Can you work these out from the model? Positions are in its coordinate system, mm. Face numbers are marked on the shaded views. Give positions to 0.01 mm unless a question says otherwise; leave off trailing zeros. Write each loop counter-clockwise with the first axis right and the second up, starting at its lowest first coordinate (ties: lowest second). Pieces come first, ordered by that corner, then holes. Notation, with made-up numbers: (66, -3) -> (112, -3) arc R11 ccw to (112, 3) -> close; hole circle Ø5 at (36, -19). An arc over 180 degrees is marked (long way). One line per item, written item: value.
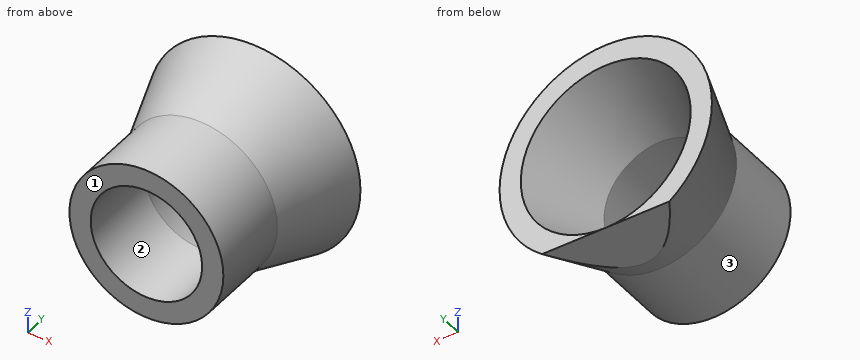
from build123d import *

# Parameters (mm, degrees)
CROQUIS2_R              = 7.25
CROQUIS2_R_2            = 5.25
SALIENTE_EXTRUIR1_DEPTH = 7.5
CORTAR_EXTRUIR1_DEPTH   = 7.5


with BuildPart() as part:
    # Croquis1 → Revolución1 (revolve)
    with BuildSketch(Plane.XY):
        Polygon((-5.25, 0), (-8, 7.5), (-10, 7.5), (-7.25, 0), align=None)
    revolve(axis=Axis((0, 7.5, 0), (0, -1, 0)))

    # Croquis2 → Saliente-Extruir1 (add)
    with BuildSketch(Plane.XZ):
        Circle(CROQUIS2_R)
        Circle(CROQUIS2_R_2, mode=Mode.SUBTRACT)
    extrude(amount=SALIENTE_EXTRUIR1_DEPTH)

    # Croquis4 → Cortar-Extruir1 (cut)
    with BuildSketch(Plane(origin=(0, 7.5, 0), x_dir=(1, 0, 0), z_dir=(0, 1, 0))):
        Polygon((-8.604100246, 8), (8.604100246, 8), (0, 12.592023512), align=None)
    extrude(amount=-CORTAR_EXTRUIR1_DEPTH, mode=Mode.SUBTRACT)


solid = part.part
1) If we section it at A-A (z = 0): Write out the boundary of the cut face in (x, y).
Answer list:
outline: (-10, 7.5) -> (-7.25, 0) -> (-7.25, -7.5) -> (-5.25, -7.5) -> (-5.25, 0) -> (-8, 7.5) -> close; (5.25, -7.5) -> (7.25, -7.5) -> (7.25, 0) -> (10, 7.5) -> (8, 7.5) -> (5.25, 0) -> close
2) Will these pins go through, and if not, where does the flat tip stop? pin 1 (8 mm diameter, centred on y = 2.5, z = 3.5, fed in from -X); pin 2 (3 mm diameter, centred on x = 6.5, y = -0.5, fed in from -Z); pin 3 (2 mm diameter, centred on y = 4.5, z = -4.5, fed in from +X).
Answer list:
pin 1: stops at x = -9.32
pin 2: stops at z = -5.25
pin 3: stops at x = 8.34
3) If we section it at B-B (y = -0.75): Write out the boundary of the cut face in (x, z), and give its area (3 significant figures).
Answer list:
outline: circle Ø14.5 at (0, 0); hole circle Ø10.5 at (0, 0)
area: 78.5 mm^2
4) We'd pull the mould along X, two halves only. Please class the marked faces 1, 2 and 3: released by +X, released by -X, zero draft, split by the parting line, or undercut.
Answer list:
face 1: zero draft
face 2: undercut
face 3: split by the parting line
5) I need wall thicknesses on L1, parallel to Z at x = 0, y = -5.25; L2, parallel to Z at x = 0.25, y = 3.25. Which ranges of each line are inside material? Lowest first, please.
Answer list:
L1: z = -7.25 to -5.25, 5.25 to 7.25
L2: z = -8 to -6.44, 6.44 to 8.44
6) If we section it at C-C (y = 4): Write out the boundary of the cut face in (x, z).
Answer list:
outline: (-3.46, -8) -> (3.46, -8) arc R8.72 ccw (long way) to start; hole circle Ø13.43 at (0, 0)
